Can you work these out from the model? Positions are in its coordinate system, mm. A direction names the side the tool comes from. Give positions to 0.01 mm unless a question says otherwise; leave off trailing zeros. Order: outer loops, then holes, each group sorted by start corner. A loop starts at its lowest first (then second) coordinate and runs counter-clockwise, first axis right, second up. Notation, with made-up numbers: M -11,0.5 L -1,0.5 A14 cw -1,12.5 Z; hole C -4,10.5 d8. An arc over 180 degrees is marked long. Answer as a JSON object with one key per item and string values.
```python
from build123d import *

# Parameters (mm, degrees)
SKETCH_1_W          = 20.7
SKETCH_1_H          = 20
EXTRUDE_1_DEPTH     = 4
SKETCH_2_W          = 4
SKETCH_2_H          = 20
EXTRUDE_2_DEPTH     = 25
SKETCH_3_R          = 2.5
CUT_EXTRUDE_1_DEPTH = 4
SKETCH_4_R          = 3
CUT_EXTRUDE_2_DEPTH = 4
CHAMFER_1_SIZE      = 6


with BuildPart() as part:
    # Эскиз1 → Бобышка-Вытянуть1 (new body)
    with BuildSketch(Plane(origin=(0, 0, 0), x_dir=(0, 0, -1), z_dir=(1, 0, 0))):
        with Locations((10.35, 10)):
            Rectangle(SKETCH_1_W, SKETCH_1_H)
    extrude(amount=EXTRUDE_1_DEPTH)

    # Эскиз2 → Бобышка-Вытянуть2 (add)
    with BuildSketch(Plane(origin=(4, 0, 0), x_dir=(0, 0, -1), z_dir=(1, 0, 0))):
        with Locations((18.7, 10)):
            Rectangle(SKETCH_2_W, SKETCH_2_H)
    extrude(amount=EXTRUDE_2_DEPTH)

    # Эскиз3 → Вырез-Вытянуть1 (cut)
    with BuildSketch(Plane.ZY):
        with Locations((-10.7, 15)):
            Circle(SKETCH_3_R)
        with Locations((-10.7, 5)):
            Circle(SKETCH_3_R)
    extrude(amount=-CUT_EXTRUDE_1_DEPTH, mode=Mode.SUBTRACT)

    # Эскиз4 → Вырез-Вытянуть2 (cut)
    with BuildSketch(Plane(origin=(0, 0, -20.7), x_dir=(-1, 0, 0), z_dir=(0, 0, -1))):
        with Locations((-21, 10)):
            Circle(SKETCH_4_R)
    extrude(amount=-CUT_EXTRUDE_2_DEPTH, mode=Mode.SUBTRACT)

    # Фаска1
    chamfer_1_edges = [part.edges().sort_by_distance(p)[0] for p in [
        (29, 0, -18.7),
        (29, 20, -18.7),
    ]]
    chamfer(chamfer_1_edges, length=CHAMFER_1_SIZE)


solid = part.part
```
1) I need wall thicknesses on L1, parallel to Y at x = 3.1, z = -10.7; L2, parallel to Y at x = 21, z = -18.55; L3, parallel to Z at x = 19, y = 14. Which ranges of each line are inside material? Lowest first, please.
Results found:
{"L1": "y = 0 to 2.5, 7.5 to 12.5, 17.5 to 20", "L2": "y = 0 to 7, 13 to 20", "L3": "z = -20.7 to -16.7"}
2) I want a section at D-D on z = -11.5. Write out the boundary of the cut face in (x, y).
Results found:
{"outline": "M 0,0 L 4,0 L 4,2.63 L 0,2.63 Z; M 0,7.37 L 4,7.37 L 4,12.63 L 0,12.63 Z; M 0,17.37 L 4,17.37 L 4,20 L 0,20 Z"}
3) I want a section at B-B on x = 21. Write out the boundary of the cut face in (y, z), and give its area (3 significant figures).
Results found:
{"outline": "M 0,-20.7 L 7,-20.7 L 7,-16.7 L 0,-16.7 Z; M 13,-20.7 L 20,-20.7 L 20,-16.7 L 13,-16.7 Z", "area": "56.0 mm²"}
4) For faces 4 (the face through (14, 10, -20.7)), 5 (the face through (4, 10, -8)), which set-ups out of +Z, -Z, +X, -X, +Y, -Y let a thin tool reach every point of the face, with its end or its side?
Results found:
{"face 4": "-Z, +X, -X, +Y, -Y", "face 5": "+Z, +X, +Y, -Y"}
5) I want a section at C-C on z = -17.25. Write out the boundary of the cut face in (x, y), and give its area (3 significant figures).
Results found:
{"outline": "M 0,0 L 23,0 L 29,6 L 29,14 L 23,20 L 0,20 Z; hole C 21,10 d6", "area": "516 mm²"}
6) I want a section at A-A on y = 10. Write out the boundary of the cut face in (x, z), and give its area (3 significant figures).
Results found:
{"outline": "M 0,-20.7 L 18,-20.7 L 18,-16.7 L 4,-16.7 L 4,0 L 0,0 Z; M 24,-20.7 L 29,-20.7 L 29,-16.7 L 24,-16.7 Z", "area": "159 mm²"}
7) I'm going to push a flat-ended pin straight in: pin 1 Ø10 at (x, y) = (10.5, 5) entering from +Z. Where does the tip first touch, or does it pass through?
Results found:
{"pin 1": "stops at z = -16.7"}
8) Thinking about a two-plate mould opening in Z: for faces 1 (the face through (29, 10, -19)), 2 (the face through (2, 13.5, -12.7)), 3 (the face through (2, 10, 0)), which applies, pulls with the +Z half, pulls with the -Z half, needs draft (parallel to the pull), parting line crosses it, or undercut?
Results found:
{"face 1": "needs draft", "face 2": "undercut", "face 3": "pulls with the +Z half"}
